Here's how the part is built. I have some questions about the finished solid (model axes, mm). Round coordinates to 2 decimals unless told otherwise and drop trailing zeros. Write each loop counter-clockwise with the first axis right and the second up, starting at its lowest first coordinate (ties: lowest second). Pieces come first, ordered by that corner, then holes. Notation, with made-up numbers: (4, 46) -> (31, 46) arc R29 ccw to (31, 69) -> close; hole circle Ø8 at (-24.75, 10.25). An arc over 180 degrees is marked (long way). Answer in a Markdown table with one row per item. Add a question column.
from build123d import *

# Parameters (mm, degrees)
SKETCH1_R           = 1.0541
SKETCH1_R_2         = 0.8001
BOSS_EXTRUDE1_DEPTH = 90
CUT_EXTRUDE2_DEPTH  = 10


with BuildPart() as part:
    # Sketch1 → Boss-Extrude1 (new body)
    with BuildSketch(Plane(origin=(0, 0, 0), x_dir=(0, 0, -1), z_dir=(1, 0, 0))):
        Circle(SKETCH1_R)
        Circle(SKETCH1_R_2, mode=Mode.SUBTRACT)
    extrude(amount=BOSS_EXTRUDE1_DEPTH)

    # Sketch3 → Cut-Extrude2 (cut)
    with BuildSketch(Plane.XY):
        with BuildLine():
            Line((1.079657865, 0.79375), (4.229657865, 0.79375))
            ThreePointArc((4.229657865, 0.79375), (5.023407865, 0), (4.229657865, -0.79375))
            Line((4.229657865, -0.79375), (1.079657865, -0.79375))
            ThreePointArc((1.079657865, -0.79375), (0.285907865, 0), (1.079657865, 0.79375))
        make_face()
    extrude(amount=-CUT_EXTRUDE2_DEPTH, mode=Mode.SUBTRACT)


solid = part.part
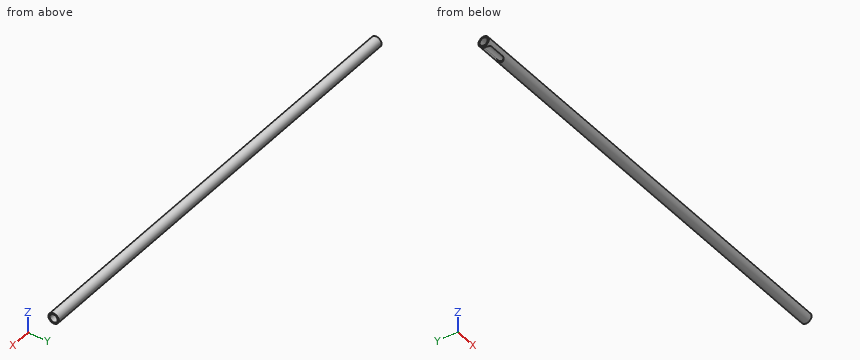
Item 1: I need wall thicknesses on line 1 along Z through (x, y) = (50.5, -0.15); line 2 along Z through (x, y) = (38, 0.05). Which ranges of each line are inside material? Lowest first, please. Write a range as from..to.
Item 2: For P1, Ø0.5, axis at x = 2.5, z = -0.5, coming from the +Y side, with a flat end and sliding along its axis, tell me the tip position at first contact or that it passes through.
Item 3: If we section it at A-A on y = 0: Please give me the cut outline in (x, z).
Item 4: If we section it at B-B on x = 13: Please give me the cut outline in (y, z), then the cut area to 3 significant figures.
Results list:
| question | item | result |
|---|---|---|
| 1 | line 1 | -1.04..-0.79, 0.79..1.04 |
| 1 | line 2 | -1.05..-0.8, 0.8..1.05 |
| 2 | P1 | y = 1.02 |
| 3 | outline | (0, -1.05) -> (0.29, -1.05) -> (0.29, -0.8) -> (0, -0.8) -> close; (0, 0.8) -> (90, 0.8) -> (90, 1.05) -> (0, 1.05) -> close; (5.02, -1.05) -> (90, -1.05) -> (90, -0.8) -> (5.02, -0.8) -> close |
| 4 | outline | circle Ø2.11 at (0, 0); hole circle Ø1.6 at (0, 0) |
| 4 | area | 1.48 mm² |
